Check sheet for the modelled part. Datum: model origin and axes. Units: mm. Give positions to 0.01 mm unless a question says otherwise; leave off trailing zeros. Order: outer loops, then holes, each group sorted by start corner. A loop starts at its lowest first (then second) coordinate and runs counter-clockwise, first axis right, second up. Notation, with made-up numbers: M 39,6.25 L 45,6.25 A25 ccw 45,22.25 Z; hole C 46,-36.5 d4. An arc over 180 degrees is marked long. Return JSON: item names as keys, results as strings. Group by question number.
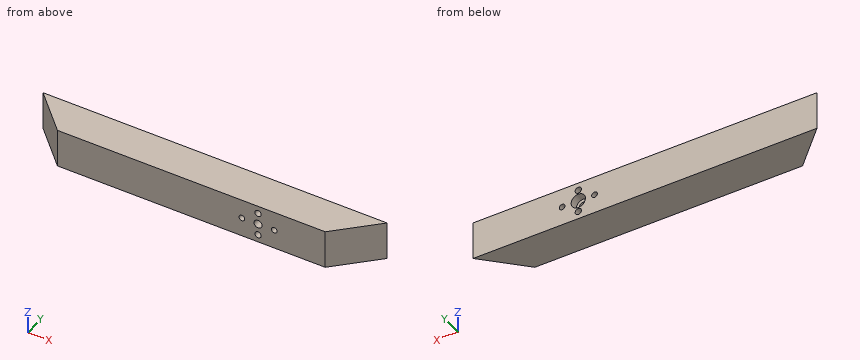
Autodesk Inventor part; units mm, degrees
ref_plane "Work Plane1" through (70, 20, 12) normal (1, 0, 0) x (0, 1, 0)
ref_plane "XZ Plane" through (0, 0, 0) normal (0, 1, 0) x (-1, 0, 0)
ref_plane "XY Plane" through (0, 0, 0) normal (0, 0, 1) x (1, 0, 0)
sketch "Skizze1" plane through (0, 0, 0) normal (0, 1, 0) x (-1, 0, 0)
  line L0 (180.5, 20) -> (-180.5, 20)
  line L1 (-180.5, 20) -> (-180.5, -20)
  line L2 (-180.5, -20) -> (180.5, -20)
  line L3 (180.5, -20) -> (180.5, 20)
  line L4 (180.5, 20) -> (-180.5, -20) construction
  line L5 (-180.5, 20) -> (180.5, -20) construction
  point P0 (0, 0)
  dimension "d0" = 361
  dimension "d1" = 40
extrude "Extrusion1" add sketch "Skizze1" along normal mid plane 40
chamfer "Fasen1" distance 40 angle 45 2 edges at (-180.5, -20, 0) (180.5, -20, 0)
sketch "Skizze2" plane through (0, 20, 0) normal (0, 1, 0) x (1, 0, 0)
  line L0 (180.5, -20) -> (180.5, 20)
  line L1 (-180.5, 20) -> (-180.5, -20)
  line L2 (180.5, 20) -> (-180.5, 20)
  line L3 (-180.5, 0) -> (180.5, 0) construction
  line L4 (-180.5, -20) -> (180.5, -20)
  line L5 (70, -20) -> (70, 20) construction
  point P0 (0, 0)
  point P1 (70, 0)
  point P2 (87, 0)
  point P3 (53, 0)
  point P4 (70, -12)
  point P5 (70, 12)
  point P6 (70, 0)
  dimension "d24" = 20
  dimension "d25" = 17
  dimension "d26" = 17
  dimension "d34" = 70
  dimension "d35" = 12
  dimension "d36" = 12
hole "Bohrung1" at (87, 20, 0) at (53, 20, 0) direction (0, -1, 0) diameter 6 end through all
hole "Hole3" at (70, 20, 0) direction (0, -1, 0) diameter 8.4 end through all counterbore diameter 15 counterbore depth 8.6
hole "Hole4" at (70, 20, 12) at (70, 20, -12) direction (0, -1, 0) diameter 6.647 end through all
ref_plane "Work Plane1" through (70, 20, 12) normal (1, 0, 0) x (0, 1, 0)
equation "\"d0\" = Laenge_Rahmen"
equation "\"d1\" = Breite_Rahmen"
equation "\"d2\" = Hoehe_Rahmen"
equation "\"d4\" = Breite_Rahmen"
equation "\"d24\" = Abstand_Bohrung_Rahmen"
equation "\"d9\" = Durchmesser_Stifte"
equation "\"Breite_Rahmen\" = 40"
equation "\"Hoehe_Rahmen\" = Breite_Rahmen"
equation "\"Breite_Bauteiltraeger\" = 239"
equation "\"Lange_Bauteiltraeger\" = Breite_Bauteiltraeger"
equation "\"Laenge_Rahmen\" = Innenmaß_Rahmen + 2 * Breite_Rahmen"
equation "\"Toleranz_Verstellung\" = 1"
equation "\"Abtand_Fuehrungsstifte\" = 34"
equation "\"Durchmesser_Stifte\" = 6"
equation "\"Abstand_Bohrung_Rahmen\" = 20"
equation "\"Exzentrizität\" = 70"
equation "\"Madenschraube_Abstand\" = 12"
properties part number "TS_Positionierungseinheit_Rahmen_int"
1) Depth check by flat-ended pin: P1, Ø6.5, axis at x = 70, z = 0, coming from the -Y side; P2, Ø1.5, axis at y = -3, z = -7.5, coming from the +X side; P3, Ø1.5, axis at y = -2, z = 15, coming from the +X side. Enter the tip coordinate at first touch or a pass-through.
2) Sectioned sample at B-B on x = 70. Record the boundary of the cut face in (y, z), then the cut area to 3 significant figures.
3) Sectioned sample at C-C on y = -14. Record the boundary of the cut face in (x, z), then the cut area to 3 significant figures.
4) Material ranges on line 1 along Z through (x, y) = (70, 7); line 2 along Z through (x, y) = (70, 16); line 3 along Z through (x, y) = (53, -4), recorded low to high.
5) Sectioned sample at A-A on z = 0. State how many separate pieces and enclosed holes the cut face has, then the cut area to 3 significant figures.
Reply:
{
 "1": {"P1": "through", "P2": "x = 158.25", "P3": "x = 159.25"},
 "2": {"outline": "M -20,-20 L 20,-20 L 20,-15.32 L -20,-15.32 Z; M -20,-8.68 L 20,-8.68 L 20,-7.5 L 11.4,-7.5 L 11.4,-4.2 L -20,-4.2 Z; M -20,4.2 L 11.4,4.2 L 11.4,7.5 L 20,7.5 L 20,8.68 L -20,8.68 Z; M -20,15.32 L 20,15.32 L 20,20 L -20,20 Z", "area": "675 mm^2"},
 "3": {"outline": "M -146.5,-20 L 146.5,-20 L 146.5,20 L -146.5,20 Z; hole C 53,0 d6; hole C 70,0 d8.4; hole C 70,-12 d6.65; hole C 70,12 d6.65; hole C 87,0 d6", "area": "11,500 mm^2"},
 "4": {"line 1": "-20 to -15.32, -8.68 to -4.2, 4.2 to 8.68, 15.32 to 20", "line 2": "-20 to -15.32, -8.68 to -7.5, 7.5 to 8.68, 15.32 to 20", "line 3": "-20 to -3, 3 to 20"},
 "5": {"separate pieces": "4", "enclosed holes": "0", "area": "12,000 mm^2"}
}
